```python
from build123d import *

# Parameters (mm, degrees)
SKETCH_1_W          = 600
SKETCH_1_H          = 600
EXTRUDE_1_DEPTH     = 4
SKETCH_2_W          = 80
SKETCH_2_H          = 150
CUT_EXTRUDE_1_DEPTH = 4
FILLET_1_R          = 15


with BuildPart() as part:
    # 草图1 → 凸台-拉伸1 (new body)
    with BuildSketch(Plane(origin=(0, 0, 0), x_dir=(1, 0, 0), z_dir=(0, 1, 0))):
        Rectangle(SKETCH_1_W, SKETCH_1_H)
    extrude(amount=EXTRUDE_1_DEPTH)

    # 草图2 → 切除-拉伸1 (cut)
    with BuildSketch(Plane.XZ):
        with Locations((260, 0)):
            Rectangle(SKETCH_2_W, SKETCH_2_H)
    cut_extrude_1 = extrude(amount=-CUT_EXTRUDE_1_DEPTH, mode=Mode.SUBTRACT)

    # 镜向1: 切除-拉伸1 across plane
    add(cut_extrude_1.mirror(Plane(origin=(0, 0, 0), x_dir=(0, 0, 1), z_dir=(1, 0, 0))), mode=Mode.SUBTRACT)

    # 圆角1
    fillet_1_edges = [part.edges().sort_by_distance(p)[0] for p in [
        (300, 2, 75),
        (300, 2, -75),
        (220, 2, -75),
        (220, 2, 75),
        (-220, 2, -75),
        (-220, 2, 75),
        (-300, 2, 75),
        (-300, 2, -75),
    ]]
    fillet(fillet_1_edges, radius=FILLET_1_R)


solid = part.part
```
CAD build for the part. Positions are in the model's coordinates, mm. A direction names the side the tool comes from. Coordinates: 2 decimals unless noted, no trailing zeros. Order: outer loops, then holes, each group sorted by start corner. A loop starts at its lowest first (then second) coordinate and runs counter-clockwise, first axis right, second up. Notation, with made-up numbers: (1.25, -32) - (5.25, -32) arc R12 cw to (5.25, -9) - close; hole circle Ø6 at (82, -37.75). An arc over 180 degrees is marked (long way). Use a Markdown table: item, result. Add a question column.
(1) Which spindle directions (+Z, -Z, +X, -X, +Y, -Y) get a long thin tool onto all of the face, cutting with end or side? Do faces 1 (the face through (-224.28, 2.03, -70.49)), 2 (the face through (-4, 0, -4)), 3 (the face through (295.72, 2.03, -79.51)). Say none if no direction does.
(2) Drill centre lines: line 1 along Z through (x, y) = (234, 3.2); line 2 along X through (y, z) = (0.9, -19); line 3 along Z through (x, y) = (-225.5, 3.5). Where is each one in solid material? Low to high. Write a range as [from, to].
(3) Saw through at A-A (y = 1.25). Give the cut face in (x, z).
(4) Saw through at B-B (z = 28.5). Give the cut face in (x, y), then the cut area to 3 significant figures.
(5) Flat gauge pin, fed straight in: pin 1 (2 mm diameter, centred on y = 2, z = -9.5, fed in from -X). Where does the tip first touch, or does it go through?
(6) Pull direction Z, two halves, no side cores. Call faces 4 (the face through (224.51, 2.03, -70.72)), 5 (the face through (-4, 4, -4)): +Z half, -Z half, draft (parallel to the pull), parting line (faces both ways), or undercut.
Solved:
| question | item | result |
|---|---|---|
| 1 | face 1 | -X, +Y, -Y |
| 1 | face 2 | +Z, -Z, +X, -X, -Y |
| 1 | face 3 | +X, +Y, -Y |
| 2 | line 1 | z = [-300, -74.97], [74.97, 300] |
| 2 | line 2 | x = [-220, 220] |
| 2 | line 3 | z = [-300, -71.61], [71.61, 300] |
| 3 | outline | (-300, -300) - (300, -300) - (300, -90) arc R15 ccw to (285, -75) - (235, -75) arc R15 cw to (220, -60) - (220, 60) arc R15 cw to (235, 75) - (285, 75) arc R15 ccw to (300, 90) - (300, 300) - (-300, 300) - (-300, 90) arc R15 ccw to (-285, 75) - (-235, 75) arc R15 cw to (-220, 60) - (-220, -60) arc R15 cw to (-235, -75) - (-285, -75) arc R15 ccw to (-300, -90) - close |
| 4 | outline | (-220, 0) - (220, 0) - (220, 4) - (-220, 4) - close |
| 4 | area | 1,760 mm² |
| 5 | pin 1 | stops at x = -220 |
| 6 | face 4 | undercut |
| 6 | face 5 | draft |
